Geometry check sheet. Reference: drawing and pictorial views, mm from the part's lowest x, y, z. A direction names the side the tool comes from. Round coordinates to 2 decimals unless told otherwise and drop trailing zeros. Write each loop counter-clockwise with the first axis right and the second up, starting at its lowest first coordinate (ties: lowest second). Pieces come first, ordered by that corner, then holes. Notation, with made-up numbers: M 67,41 L 74,41 A22 cw 74,65 Z; hole C 75,88.5 d10. An arc over 180 degrees is marked long. Use a Markdown table: item, result. Add a question column.
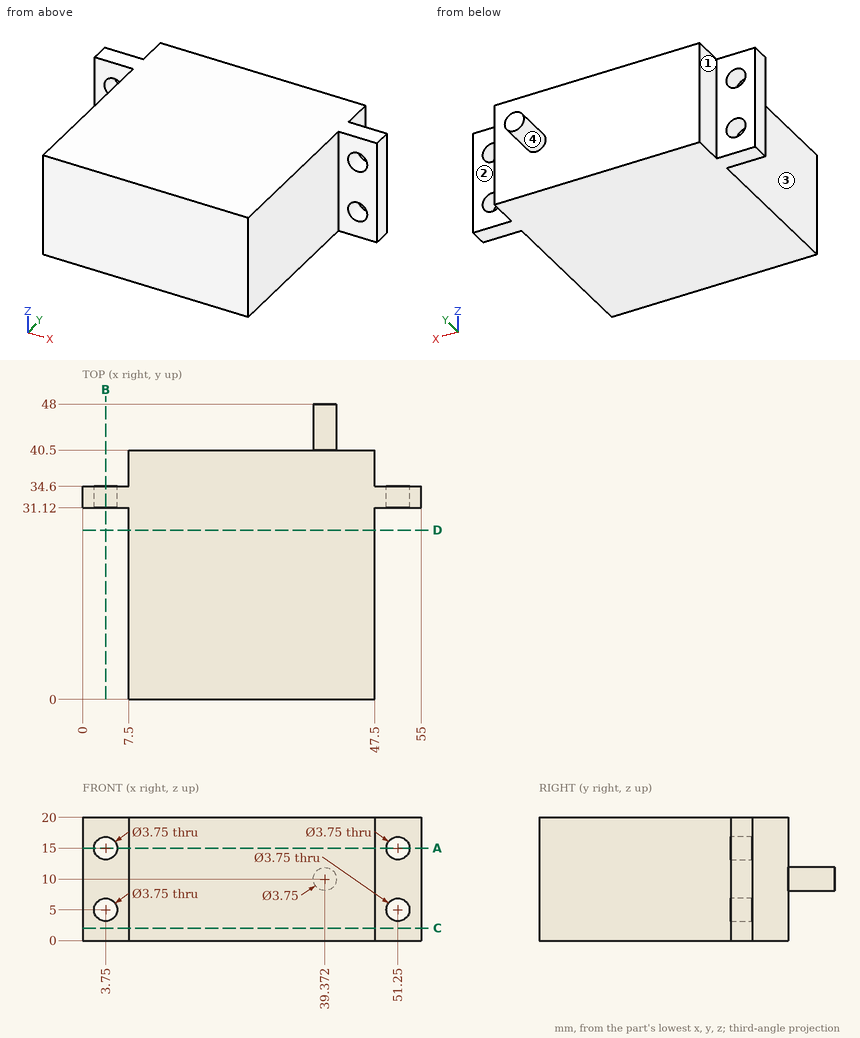
1. Depth check by flat-ended pin: pin 1 Ø4 at (x, z) = (52.5, 6) entering from +Y; pin 2 Ø4.5 at (x, z) = (3.75, 5) entering from -Y; pin 3 Ø10 at (y, z) = (23, 13.5) entering from +X. Enter the tip coordinate at first touch or a pass-through.
2. Cross-section at B-B on x = 3.75. Enter the section's corners in (y, z) (1 decimal).
3. Access from +Z, -Z, +X, -X, +Y, -Y to the whole of each face (thin tool, end or side, straight path). Record for the marked faces 1, 2, 3 and 4.
4. Cross-section at A-A on z = 15. Enter the section's corners in (x, y) (1 decimal).
5. Cross-section at C-C on z = 2. Enter the section's corners in (x, y), plus the area to 3 significant figures.
6. Cross-section at D-D on y = 27.5. Enter the section's corners in (x, z), plus the area to 3 significant figures.
7. Scan lines: line 1 along X through (y, z) = (32, 15) (1 decimal); line 2 along Y through (x, z) = (21.5, 1.5); line 3 along X through (y, z) = (12, 7.25). Record each from-to range of solid material in increasing order. Write a range as from..to.
Answer:
| question | item | result |
|---|---|---|
| 1 | pin 1 | stops at y = 34.6 |
| 1 | pin 2 | stops at y = 31.12 |
| 1 | pin 3 | stops at x = 47.5 |
| 2 | outline | M 31.1,0 L 34.6,0 L 34.6,3.1 L 31.1,3.1 Z; M 31.1,6.9 L 34.6,6.9 L 34.6,13.1 L 31.1,13.1 Z; M 31.1,16.9 L 34.6,16.9 L 34.6,20 L 31.1,20 Z |
| 3 | face 1 | +Z, -Z, -X, +Y |
| 3 | face 2 | +Z, -Z, +X, +Y |
| 3 | face 3 | +Z, -Z, -X, -Y |
| 3 | face 4 | +Y |
| 4 | outline | M 0,31.1 L 1.9,31.1 L 1.9,34.6 L 0,34.6 Z; M 5.6,31.1 L 7.5,31.1 L 7.5,0 L 47.5,0 L 47.5,31.1 L 49.4,31.1 L 49.4,34.6 L 47.5,34.6 L 47.5,40.5 L 7.5,40.5 L 7.5,34.6 L 5.6,34.6 Z; M 53.1,31.1 L 55,31.1 L 55,34.6 L 53.1,34.6 Z |
| 5 | outline | M 0,31.12 L 7.5,31.12 L 7.5,0 L 47.5,0 L 47.5,31.12 L 55,31.12 L 55,34.6 L 47.5,34.6 L 47.5,40.5 L 7.5,40.5 L 7.5,34.6 L 0,34.6 Z |
| 5 | area | 1,670 mm^2 |
| 6 | outline | M 7.5,0 L 47.5,0 L 47.5,20 L 7.5,20 Z |
| 6 | area | 800 mm^2 |
| 7 | line 1 | x = 0..1.9, 5.6..49.4, 53.1..55 |
| 7 | line 2 | y = 0..40.5 |
| 7 | line 3 | x = 7.5..47.5 |
